For this review, take the finished solid that the model builds, in its own axes (mm). A direction names the side the tool comes from. Round coordinates to 2 decimals unless told otherwise and drop trailing zeros. Order: outer loops, then holes, each group sorted by start corner. A loop starts at its lowest first (then second) coordinate and runs counter-clockwise, first axis right, second up.
from build123d import *
from OCP.BRepFilletAPI import BRepFilletAPI_MakeChamfer

# Parameters (mm, degrees)
SKETCH1_W                = 114
SKETCH1_H                = 43.5
BOSS_EXTRUDE1_DEPTH      = 3.7
SKETCH2_W                = 4.4
SKETCH2_H                = 43.5
BOSS_EXTRUDE2_DEPTH      = 3
CHAMFER1_SIZE            = 2
CHAMFER1_SIZE2           = 5.494954839
CUT_EXTRUDE1_DEPTH       = 7.5
BOSS_EXTRUDE3_DEPTH      = 3.25
BOSS_EXTRUDE3_DEPTH_BACK = 46.75
SKETCH6_W                = 4.4
SKETCH6_H                = 6.7
FILLET2_R                = 1
CHAMFER2_SIZE            = 1
CHAMFER2_SIZE2           = 2.747477419


with BuildPart() as part:
    # Sketch1 → Boss-Extrude1 (new body)
    with BuildSketch(Plane(origin=(0, 0, 0), x_dir=(1, 0, 0), z_dir=(0, 1, 0))):
        with Locations((57, 21.75)):
            Rectangle(SKETCH1_W, SKETCH1_H)
    extrude(amount=BOSS_EXTRUDE1_DEPTH)

    # Sketch2 → Boss-Extrude2 (add)
    with BuildSketch(Plane(origin=(0, 3.7, 0), x_dir=(1, 0, 0), z_dir=(0, 1, 0))):
        with Locations((111.8, 21.75)):
            Rectangle(SKETCH2_W, SKETCH2_H)
    extrude(amount=BOSS_EXTRUDE2_DEPTH)

    # Chamfer1
    chamfer1_edges = [part.edges().sort_by_distance(p)[0] for p in [
        (0, 1.85, -43.5),
        (0, 1.85, 0),
    ]]
    chamfer1_side = [part.faces().sort_by_distance(p)[0] for p in [
        (0, 1.85, -21.75),
    ]]
    chamfer(chamfer1_edges, length=CHAMFER1_SIZE, length2=CHAMFER1_SIZE2, reference=chamfer1_side[0])

    # Sketch3 → Cut-Extrude1 (cut)
    with BuildSketch(Plane(origin=(0, 3.7, 0), x_dir=(1, 0, 0), z_dir=(0, 1, 0))):
        Polygon((4, 6.439957255), (23.046483703, 19.75), (4, 19.75), align=None)
        Polygon((27.4, 4), (27.4, 17.91240495), (7.491544466, 4), align=None)
        Polygon((23.046483703, 23.75), (4, 37.060042745), (4, 23.75), align=None)
        Polygon((27.4, 25.58759505), (27.4, 39.5), (7.491544466, 39.5), align=None)
        Polygon((31.4, 25.58759505), (51.308455534, 39.5), (31.4, 39.5), align=None)
        Polygon((52.8, 23.75), (52.8, 35.66240495), (35.753516297, 23.75), align=None)
        Polygon((52.8, 7.83759505), (52.8, 19.75), (35.753516297, 19.75), align=None)
        Polygon((31.4, 4), (51.308455534, 4), (31.4, 17.91240495), align=None)
        Polygon((73.846483703, 19.75), (56.8, 19.75), (56.8, 7.83759505), align=None)
        Polygon((78.2, 17.91240495), (58.291544466, 4), (78.2, 4), align=None)
        Polygon((56.8, 35.66240495), (56.8, 23.75), (73.846483703, 23.75), align=None)
        Polygon((78.2, 39.5), (58.291544466, 39.5), (78.2, 25.58759505), align=None)
        Polygon((102.108455534, 39.5), (82.2, 39.5), (82.2, 25.58759505), align=None)
        Polygon((105.6, 23.75), (105.6, 37.060042745), (86.553516297, 23.75), align=None)
        Polygon((105.6, 19.75), (86.553516297, 19.75), (105.6, 6.439957255), align=None)
        Polygon((82.2, 17.91240495), (82.2, 4), (102.108455534, 4), align=None)
    extrude(amount=-CUT_EXTRUDE1_DEPTH, mode=Mode.SUBTRACT)

    # Sketch6 → Boss-Extrude3 (add, two sides: drawn at the far end of the back side and taken through both)
    with BuildSketch(Plane.XY.offset(-BOSS_EXTRUDE3_DEPTH_BACK)):
        with Locations((111.8, 3.35)):
            Rectangle(SKETCH6_W, SKETCH6_H)
    extrude(amount=BOSS_EXTRUDE3_DEPTH + BOSS_EXTRUDE3_DEPTH_BACK)

    # Fillet2
    fillet2_edges = [part.edges().sort_by_distance(p)[0] for p in [
        (114, 6.7, -21.75),
        (109.6, 6.7, -21.75),
    ]]
    fillet(fillet2_edges, radius=FILLET2_R)

    # Chamfer2: one chamfer whose edges measure the first distance from different faces: ONE call of the kernel's chamfer builder (chamfer() names one face for all edges)
    chamfer2_edges_1 = [part.edges().sort_by_distance(p)[0] for p in [
        (0, 3.7, -21.75),
    ]]
    chamfer2_side_1 = [part.faces().sort_by_distance(p)[0] for p in [
        (0, 1.85, -21.75),
    ]]
    chamfer2_edges_2 = [part.edges().sort_by_distance(p)[0] for p in [
        (2.747477419, 3.7, -1),
    ]]
    chamfer2_side_2 = [part.faces().sort_by_distance(p)[0] for p in [
        (2.747477419, 1.85, -1),
    ]]
    chamfer2_edges_3 = [part.edges().sort_by_distance(p)[0] for p in [
        (2.747477419, 3.7, -42.5),
    ]]
    chamfer2_side_3 = [part.faces().sort_by_distance(p)[0] for p in [
        (2.747477419, 1.85, -42.5),
    ]]
    chamfer2 = BRepFilletAPI_MakeChamfer(part.part.solid().wrapped)
    for e in chamfer2_edges_1:
        chamfer2.Add(CHAMFER2_SIZE, CHAMFER2_SIZE2, e.wrapped, chamfer2_side_1[0].wrapped)  # the first distance lies on this face
    for e in chamfer2_edges_2:
        chamfer2.Add(CHAMFER2_SIZE, CHAMFER2_SIZE2, e.wrapped, chamfer2_side_2[0].wrapped)  # the first distance lies on this face
    for e in chamfer2_edges_3:
        chamfer2.Add(CHAMFER2_SIZE, CHAMFER2_SIZE2, e.wrapped, chamfer2_side_3[0].wrapped)  # the first distance lies on this face
    add(Compound.cast(chamfer2.Shape()), mode=Mode.REPLACE)


solid = part.part
(1) Add section C-C on y = 1.5. Count the separate pieces of the cut face and the enclosed holes in it, plus the area to 3 significant figures.
(2) Wall thickness on L1, parallel to Z at x = 73, y = 3; L2, parallel to Z at x = 64, y = 0.5; L3, parallel to Y at x = 12, z = -11.5: over which ranges is each line inside the solid? List them lowest first.
(3) Clearance check with flat-ended pins moving along their axes: P1, Ø3, axis at x = 18, y = 2, coming from the -Z side; P2, Ø3, axis at x = 98.5, y = 1, coming from the +Z side; P3, Ø6, axis at x = 59, z = -38.5, coming from the +Y side; P4, Ø1.5, axis at x = 58.5, y = 5.5, coming from the -Z side. State where each tip first meets the part, or that it passes through.
(4) Tool access review of faces 5 (the face through (57, 2, -43.5)), 6 (the face through (55, 3.7, -22)), 7 (the face through (41, 2, -4)), 8 (the face through (2.786, 1.331, -0.986)): name each direction out of +Z, -Z, +X, -X, +Y, -Y from which nothing blocks a thin tool from reaching the whole face with its end or side.
(5) Add section B-B on x = 85. Give the boundary of the cut face in (y, z), plus the area to 3 significant figures.
(6) Add section A-A on x = 68. Give the boundary of the cut face in (y, z).
(7) Draft analysis for pull direction Z (two halves, no side actions). For faces 1 (the face through (56, 0, -22)), 2 (the face through (112, 3, 3.25)), 3 (the face through (65.443, 1.876, -29.623)), 4 (the face through (112, 3, -46.75)), state which applies: pulls with the +Z half, pulls with the -Z half, needs draft (parallel to the pull), parting line crosses it, or undercut.
Here are the results:
1. separate pieces: 1
1. enclosed holes: 16
1. area: 2,960 mm2
2. L1: z = -43.5 to -39.5, -29.22 to -24.34, -23.75 to -19.75, -19.16 to -14.28, -4 to 0
2. L2: z = -43.5 to -39.5, -35.51 to -30.63, -23.75 to -19.75, -12.87 to -7.99, -4 to 0
2. L3: y = 0 to 3.7
3. P1: stops at z = -43.5
3. P2: stops at z = 0
3. P3: stops at y = 3.7
3. P4: passes through
4. face 5: -Z, -X, +Y, -Y
4. face 6: +Z, -Z, -X, +Y
4. face 7: +Y, -Y
4. face 8: +Z, -X, +Y, -Y
5. outline: (0, -43.5) - (3.7, -43.5) - (3.7, -39.5) - (0, -39.5) - close; (0, -27.54) - (3.7, -27.54) - (3.7, -15.96) - (0, -15.96) - close; (0, -4) - (3.7, -4) - (3.7, 0) - (0, 0) - close
5. area: 72.5 mm2
6. outline: (0, -43.5) - (3.7, -43.5) - (3.7, -39.5) - (0, -39.5) - close; (0, -32.72) - (3.7, -32.72) - (3.7, -27.84) - (0, -27.84) - close; (0, -23.75) - (3.7, -23.75) - (3.7, -19.75) - (0, -19.75) - close; (0, -15.66) - (3.7, -15.66) - (3.7, -10.78) - (0, -10.78) - close; (0, -4) - (3.7, -4) - (3.7, 0) - (0, 0) - close
7. face 1: needs draft
7. face 2: pulls with the +Z half
7. face 3: undercut
7. face 4: pulls with the -Z half
